from build123d import *

# Parameters (mm, degrees)
CROQUIS1_W              = 30
CROQUIS1_H              = 30
CROQUIS1_R              = 3
SALIENTE_EXTRUIR1_DEPTH = 5
CROQUIS2_R              = 9
CORTAR_EXTRUIR1_DEPTH   = 5


with BuildPart() as part:
    # Croquis1 → Saliente-Extruir1 (new body)
    with BuildSketch(Plane.XY):
        Rectangle(CROQUIS1_W, CROQUIS1_H)
        with Locations((-11, 11)):
            Circle(CROQUIS1_R, mode=Mode.SUBTRACT)
        with Locations(Location((11, 11, 0), (0, 0, 180))):
            Circle(CROQUIS1_R, mode=Mode.SUBTRACT)
    extrude(amount=SALIENTE_EXTRUIR1_DEPTH)

    # Croquis2 → Cortar-Extruir1 (cut)
    with BuildSketch(Plane.XY.offset(5)):
        Circle(CROQUIS2_R)
    extrude(amount=-CORTAR_EXTRUIR1_DEPTH, mode=Mode.SUBTRACT)


solid = part.part
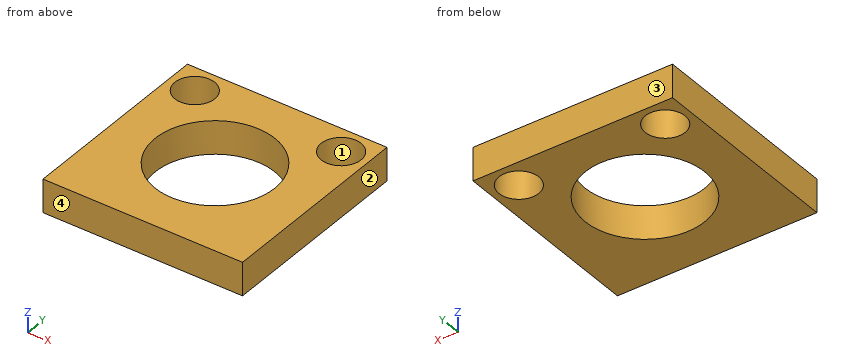
Can you work these out from the model? Positions are in its coordinate system, mm. Face numbers are marked on the shaded views. Coordinates: 2 decimals unless noted, no trailing zeros. Write each loop counter-clockwise with the first axis right and the second up, starting at its lowest first coordinate (ties: lowest second). Pieces come first, ordered by that corner, then holes. Notation, with made-up numbers: (1, 79) -> (55, 79) arc R21 cw to (55, 107) -> close; hole circle Ø8 at (41, -8). An arc over 180 degrees is marked (long way). Write each question's results on one line, items separated by ' | '. Start each with the question number.
Item 1: If we section it at A-A, the plane y = 0: Write out the boundary of the cut face in (x, z), and give its area (3 significant figures).
Item 2: If we section it at B-B, the plane z = 3.8: Write out the boundary of the cut face in (x, y).
Item 3: If we section it at D-D, the plane y = 11: Write out the boundary of the cut face in (x, z).
Item 4: Please list where these lines run through material, in increasing order: probe 1 along Y at (x, z) = (-11, 3.1); probe 2 along Y at (x, z) = (0, 1.25); probe 3 along X at (y, z) = (3.5, 0.5).
Item 5: I'm going to push a flat-ended pin straight in: P1, Ø5, axis at x = 11, y = 11, coming from the -Z side. Where does the tip first touch, or does it pass through?
Item 6: Thinking about a two-plate mould opening in Y: for the marked faces 1, 2, 3 and 4, which applies, released by +Y, released by -Y, zero draft, split by the parting line, or undercut?
Answer block:
1) outline: (-15, 0) -> (-9, 0) -> (-9, 5) -> (-15, 5) -> close; (9, 0) -> (15, 0) -> (15, 5) -> (9, 5) -> close | area: 60.0 mm²
2) outline: (-15, -15) -> (15, -15) -> (15, 15) -> (-15, 15) -> close; hole circle Ø6 at (-11, 11); hole circle Ø18 at (0, 0); hole circle Ø6 at (11, 11)
3) outline: (-15, 0) -> (-14, 0) -> (-14, 5) -> (-15, 5) -> close; (-8, 0) -> (8, 0) -> (8, 5) -> (-8, 5) -> close; (14, 0) -> (15, 0) -> (15, 5) -> (14, 5) -> close
4) probe 1: -15 to 8, 14 to 15 | probe 2: -15 to -9, 9 to 15 | probe 3: -15 to -8.29, 8.29 to 15
5) P1: through
6) face 1: undercut | face 2: zero draft | face 3: released by +Y | face 4: released by -Y
